Input: part model. Units: mm. Frame: model coordinates. A direction names the side the tool comes from. Coordinates: 2 decimals unless noted, no trailing zeros. Write each loop counter-clockwise with the first axis right and the second up, starting at its lowest first coordinate (ties: lowest second). Pieces come first, ordered by that corner, then holes. Notation, with made-up numbers: M -30.5,-33 L -1.5,-33 A11 cw -1.5,-14 Z; hole C 63.25,-16 d11. An arc over 180 degrees is marked long. Use CSV: the item, a comma, the result in double quotes.
Autodesk Inventor part; units mm, degrees
ref_plane "YZ Plane" through (0, 0, 0) normal (1, 0, 0) x (0, 1, 0)
ref_plane "XZ Plane" through (0, 0, 0) normal (0, 1, 0) x (-1, 0, 0)
ref_plane "XY Plane" through (0, 0, 0) normal (0, 0, 1) x (1, 0, 0)
sketch "Sketch1" plane through (0, 0, 0) normal (0, 1, 0) x (-1, 0, 0)
  line L0 (0, 0) -> (25, 0)
  line L1 (25, 0) -> (25, -165)
  line L2 (25, -165) -> (0, -165)
  line L3 (0, -165) -> (0, 0)
  dimension "d0" = 25
  dimension "d1" = 165
extrude "Extrusion1" add sketch "Sketch1" along normal blind 3
sketch "Sketch2" plane through (0, 3, 0) normal (0, 1, 0) x (1, 0, 0)
  line L0 (-25, 165) -> (-25, 0)
  line L1 (0, 0) -> (0, 165)
  line L2 (-25, 0) -> (0, 0)
  line L3 (0, 0) -> (0, 7)
  line L4 (0, 7) -> (-25, 7)
  line L5 (-25, 7) -> (-25, 0)
  line L6 (0, 165) -> (-25, 165)
  line L7 (-25, 165) -> (0, 165)
  line L8 (0, 165) -> (0, 158)
  line L9 (0, 158) -> (-25, 158)
  line L10 (-25, 158) -> (-25, 165)
  dimension "d4" = 7
  dimension "d5" = 7
extrude "Extrusion2" add sketch "Sketch2" along normal blind 22 contours L6 L1 L9 L0 | L4 L1 L2 L0
sketch "Sketch3" plane through (-25, 0, 0) normal (0, 0, 1) x (1, 0, 0)
  point P0 (25, 0)
sketch "Sketch4" plane through (-25, 0, 0) normal (0, 0, 1) x (1, 0, 0)
  line L0 (25, 25) -> (0, 25) construction
  line L1 (25, 0) -> (0, 25) construction
  circle A0 centre (12.5, 12.5) radius 6.5
  dimension "d8" = 13
extrude "Extrusion3" cut sketch "Sketch4" against normal blind 5
sketch "Sketch5" plane through (0, 0, -165) normal (0, 0, -1) x (-1, 0, 0)
  circle A0 centre (12.5, 12.5) radius 6.5
  circle A1 centre (12.5, 12.5) radius 6.5
  point P0 (0, 0)
extrude "Extrusion4" cut sketch "Sketch5" against normal blind 5
sketch "Sketch6" plane through (-25, 0, 0) normal (0, 0, 1) x (1, 0, 0)
  circle A0 centre (12.5, 12.5) radius 6.5
  circle A1 centre (12.5, 12.5) radius 5
  point P0 (25, 0)
  dimension "d13" = 10
extrude "Extrusion5" cut sketch "Sketch6" against normal blind 165 contours A1
sketch "Sketch7" plane through (-25, 3, -158) normal (0, 0, 1) x (1, 0, 0)
  line L0 (25, 0) -> (25, 22) construction
  line L1 (0, 0) -> (0, 22) construction
  point P0 (25, -3)
sketch "Sketch8" plane through (-25, 3, -158) normal (0, 0, 1) x (1, 0, 0)
  circle A0 centre (12.5, 9.5) radius 5
  point P0 (25, -3)
sketch "Sketch9" plane through (0, 3, 0) normal (0, 1, 0) x (1, 0, 0)
  line L0 (-25, 158) -> (0, 158)
  line L1 (0, 7) -> (-25, 7)
  line L2 (-25, 158) -> (-20, 158)
  line L3 (-20, 158) -> (-20, 7)
  line L4 (-20, 7) -> (-25, 7)
  line L5 (-25, 7) -> (-25, 158)
  line L6 (0, 0) -> (0, 7)
  line L7 (0, 7) -> (-5, 7)
  line L8 (-5, 7) -> (-5, 158)
  line L9 (-5, 158) -> (0, 158)
  line L10 (0, 158) -> (0, 7)
  dimension "d16" = 5
  dimension "d17" = 5
extrude "Extrusion6" add sketch "Sketch9" along normal blind 7.5 contours L0 L3 L1 L5 | L0 L10 L1 L8
fillet "Fillet1" radius 2 2 edges at (-5, 10.5, -82.5) (-20, 10.5, -82.5)
sketch "Sketch10" plane through (0, 0, 0) normal (1, 0, 0) x (0, 0, -1)
  line L0 (165, 0) -> (165, 25)
  line L1 (0, 0) -> (165, 0)
  line L2 (165, 0) -> (165, 3)
  line L3 (165, 3) -> (0, 3)
  line L4 (0, 3) -> (0, 0)
  dimension "d21" = 3
extrude "Extrusion7" add sketch "Sketch10" along normal blind 45
sketch "Sketch11" plane through (0, 3, 0) normal (0, 1, 0) x (1, 0, 0)
  line L0 (45, 165) -> (45, 0) construction
  line L1 (0, 165) -> (-25, 165) construction
  line L2 (45, 82.5) -> (3, 82.5) construction
  circle A0 centre (24, 82.5) radius 21 construction
  circle A1 centre (24, 124.5) radius 21 construction
  circle A2 centre (24, 124.5) radius 21
  circle A3 centre (24, 82.5) radius 21
  circle A4 centre (24, 40.5) radius 21
  circle A5 centre (24, 40.5) radius 19.325
  circle A6 centre (24, 82.5) radius 19.325
  circle A7 centre (24, 124.5) radius 19.325
  point P0 (0, 0)
  dimension "d24" = 42
  dimension "d25" = 38.65
  dimension "d26" = 38.65
  dimension "d27" = 38.65
extrude "Extrusion8" add sketch "Sketch11" along normal blind 45
sketch "Sketch12" plane through (0, 3, 0) normal (0, 1, 0) x (1, 0, 0)
  point P0 (0, 0)
sketch "Sketch13" plane through (0, 3, 0) normal (0, 1, 0) x (1, 0, 0)
  line L0 (45, 40.5) -> (45, 0)
  line L1 (0, 0) -> (0, 165)
  line L2 (45, 0) -> (0, 0)
  line L3 (0, 0) -> (0, 16)
  line L4 (0, 16) -> (45, 16)
  line L5 (45, 16) -> (45, 0)
  line L6 (45, 165) -> (45, 124.5)
  line L7 (0, 165) -> (45, 165)
  line L8 (45, 165) -> (45, 149)
  line L9 (45, 149) -> (0, 149)
  line L10 (0, 149) -> (0, 165)
  dimension "d30" = 16
  dimension "d31" = 16
extrude "Extrusion9" add sketch "Sketch13" along normal blind 22
sketch "Sketch14" plane through (45, 0, 0) normal (1, 0, 0) x (0, 0, -1)
  line L0 (0, 25) -> (16, 25) construction
  line L1 (8, 25) -> (8, 21.5) construction
  line L2 (14.125, 23.125) -> (1.875, 23.125)
  line L3 (1.875, 23.125) -> (1.875, 19.875)
  line L4 (1.875, 19.875) -> (14.125, 19.875)
  line L5 (14.125, 19.875) -> (14.125, 23.125)
  line L6 (14.125, 23.125) -> (1.875, 19.875) construction
  line L7 (1.875, 23.125) -> (14.125, 19.875) construction
  point P0 (0, 0)
  dimension "d35" = 3.5
  dimension "d36" = 12.25
  dimension "d37" = 3.25
sketch "Sketch15" plane through (45, 0, 0) normal (1, 0, 0) x (0, 0, -1)
  line L0 (149, 25) -> (165, 25) construction
  line L1 (157, 25) -> (157, 21.5) construction
  line L2 (163.125, 23.125) -> (150.875, 23.125)
  line L3 (150.875, 23.125) -> (150.875, 19.875)
  line L4 (150.875, 19.875) -> (163.125, 19.875)
  line L5 (163.125, 19.875) -> (163.125, 23.125)
  line L6 (163.125, 23.125) -> (150.875, 19.875) construction
  line L7 (150.875, 23.125) -> (163.125, 19.875) construction
  point P0 (0, 0)
  dimension "d38" = 3.5
  dimension "d39" = 12.25
  dimension "d40" = 3.25
extrude "Extrusion10" cut sketch "Sketch14" against normal blind 40
extrude "Extrusion11" cut sketch "Sketch15" against normal blind 40
sketch "Sketch16" plane through (0, 25, 0) normal (0, 1, 0) x (1, 0, 0)
  line L0 (45, 0) -> (45, 16) construction
  line L1 (45, 8) -> (20, 8) construction
  circle A0 centre (20, 8) radius 0.75 construction
  circle A1 centre (20, 8) radius 0.75
  point P0 (0, 0)
  dimension "d45" = 25
  dimension "d46" = 1.5
extrude "Extrusion12" cut sketch "Sketch16" against normal blind 25
sketch "Sketch17" plane through (0, 25, 0) normal (0, 1, 0) x (1, 0, 0)
  point P0 (0, 0)
sketch "Sketch18" plane through (0, 25, 0) normal (0, 1, 0) x (1, 0, 0)
  point P0 (0, 0)
sketch "Sketch19" plane through (0, 25, 0) normal (0, 1, 0) x (1, 0, 0)
  point P0 (0, 0)
sketch "Sketch20" plane through (0, 25, 0) normal (0, 1, 0) x (1, 0, 0)
  line L0 (0, 149) -> (45, 149) construction
  line L1 (45, 0) -> (45, 165) construction
  line L2 (45, 149) -> (45, 165) construction
  line L3 (45, 157) -> (20, 157) construction
  circle A0 centre (20, 157) radius 0.75
  point P0 (0, 0)
  dimension "d49" = 25
  dimension "d50" = 1.5
extrude "Extrusion13" cut sketch "Sketch20" against normal blind 25
sketch "Sketch21" plane through (-25, 0, -165) normal (-1, 0, 0) x (0, 0, 1)
  point P0 (165, 0)
sketch "Sketch22" plane through (-25, 0, -165) normal (-1, 0, 0) x (0, 0, 1)
  line L0 (158, 8.5) -> (7, 8.5) construction
  line L1 (82.5, 8.5) -> (82.5, 6.5) construction
  circle A0 centre (82.5, 6.5) radius 0.5
  point P0 (165, 0)
  dimension "d53" = 2
  dimension "d54" = 1
extrude "Extrusion14" cut sketch "Sketch22" against normal blind 5.25
fillet "Fillet2" radius 1 1 edges at (-25, 6.5, -83)
sketch "Sketch23" plane through (-25, 0, -165) normal (-1, 0, 0) x (0, 0, 1)
  circle A0 centre (82.5, 9.5843) radius 0.5
  point P0 (165, 0)
  dimension "d58" = 1
extrude "Extrusion15" cut sketch "Sketch23" against normal blind 5.25
sketch "Sketch24" plane through (0, 48, 0) normal (0, 1, 0) x (1, 0, 0)
  line L0 (0, 0) -> (48.5926, 0)
  line L1 (48.5926, 0) -> (48.5926, 173.5031)
  line L2 (48.5926, 173.5031) -> (0, 173.5031)
  line L3 (0, 173.5031) -> (0, 0)
properties part number "rearAxelHolder 11-28"
1. Section D-D (z = -113). Return loops of the section in (x, y).
Resolved:
outline,"M -25,0 L 45,0 L 45,3 L 41.57,3 L 41.57,48 L 39.53,48 L 39.53,3 L 8.47,3 L 8.47,48 L 6.43,48 L 6.43,3 L 0,3 L 0,10.5 L -3,10.5 A2 ccw -5,8.5 L -5,3 L -20,3 L -20,8.5 A2 ccw -22,10.5 L -25,10.5 Z"
2. Contact query for flat-ended pins moving along their axis: pin 1 Ø9 at (x, y) = (-12.5, 12.5) entering from -Z; pin 2 Ø8 at (x, z) = (21.5, -8.5) entering from +Y; pin 3 Ø16.5 at (x, z) = (-12.5, -60.5) entering from +Y; pin 4 Ø3 at (y, z) = (15, -90) entering from +X. Output: stop coordinate, or through.
Resolved:
pin 1,"passes through"
pin 2,"stops at y = 25"
pin 3,"stops at y = 10.06"
pin 4,"stops at x = 44.12"
3. Section B-B (x = -12.5). Return loops of the section in (y, z), then the cut area to 3 significant figures.
Resolved:
outline,"M 0,-165 L 6,-165 L 6,-160 L 7.5,-160 L 7.5,-158 L 3,-158 L 3,-7 L 7.5,-7 L 7.5,-5 L 6,-5 L 6,0 L 0,0 Z; M 17.5,-160 L 19,-160 L 19,-165 L 25,-165 L 25,-158 L 17.5,-158 Z; M 17.5,-7 L 25,-7 L 25,0 L 19,0 L 19,-5 L 17.5,-5 Z"
area,"633 mm^2"
4. Material intervals for line 1 (X direction, y = 23.65, z = -8); line 2 (Z direction, x = 1.5, y = 7); line 3 (X direction, y = 7.5, z = -153), sorted ascending. Write a range as [from, to].
Resolved:
line 1,"x = [0, 19.25], [20.75, 45]"
line 2,"z = [-165, -149], [-16, 0]"
line 3,"x = [-25, -20], [-5, 45]"
5. Access query for faces 1 (the flat face through (-12, 19, -158)), 2 (the flat face through (25, 21, -14.125)), 3 (the flat face through (0, 18, -153)), 4 (the flat face through (17, 25, -157)). Directions: +Z, -Z, +X, -X, +Y, -Y. A direction counts if a zero-diameter tool reaches every point of the face in a straight line with its end or side. Return the directions, or none.
Resolved:
face 1,"+Y"
face 2,"+X"
face 3,"-X, +Y"
face 4,"-Z, +X, -X, +Y"
6. Mould query, pull axis Z, two halves, no side actions, for faces 5 (the flat face through (-14.4, 7.7, -160)), 6 (the flat face through (22, 14, -16)), 7 (the flat face through (-25, 4, -81)), 8 (the flat face through (5, 22, -8)). Classes: pulls with the +Z half, pulls with the -Z half, needs draft (parallel to the pull), parting line crosses it, or undercut.
Resolved:
face 5,"pulls with the -Z half"
face 6,"undercut"
face 7,"needs draft"
face 8,"undercut"
